The listing builds one solid part. Answer for the finished solid, in the listing's coordinates (mm). Coordinates: 2 decimals unless noted, no trailing zeros. Order: outer loops, then holes, each group sorted by start corner. A loop starts at its lowest first (then second) coordinate and runs counter-clockwise, first axis right, second up. Notation, with made-up numbers: M -9,-26.5 L 36,-26.5 A24 ccw 36,12.5 Z; hole C 52.25,17.25 d3. An arc over 180 degrees is marked long. One line per item, written item: value. Start each with the question number.
Q1. Straight lines are drawn through the part: line 1 along Z through (x, y) = (366.5, 8.25); line 2 along X through (y, z) = (10.75, -336); line 3 along Z through (x, y) = (234.5, 7). For each, find the intervals that lie inside material, in ascending order. Write a range as [from, to].
Q2. The part is cut by section C-C on x = 143.5. Give the vertices of the cut face in (y, z).
Q3. The part is cut by section B-B on z = -556. Give the vertices of the cut face in (x, y), then the cut area to 3 significant figures.
Q4. Each of these flat-tipped pins is pushed along its axis until it touches: pin 1 Ø1 at (x, y) = (110.5, 2) entering from +Z; pin 2 Ø3 at (x, y) = (250, 5) entering from +Z; pin 3 Ø2 at (x, y) = (98, 1.5) entering from -Z. Where does it stop, or does it pass through?
Q5. The part is cut by section A-A on y = 9. Give the vertices of the cut face in (x, z).
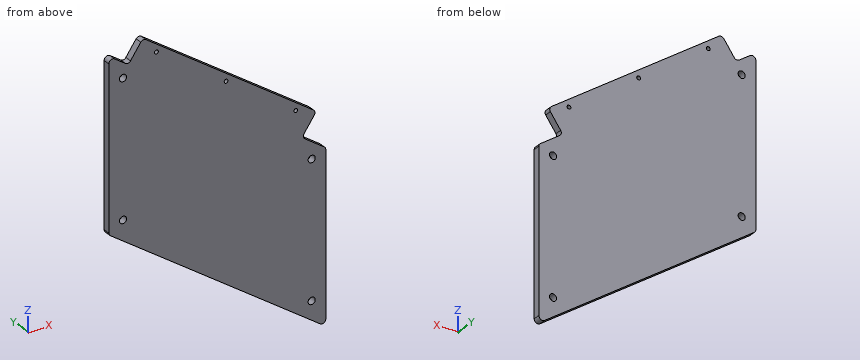
```python
from build123d import *

# Parameters (mm, degrees)
BOSS_EXTRUDE1_DEPTH = 12.7
CUT_EXTRUDE1_DEPTH  = 742.687355867
SKETCH3_R           = 3.3782
SKETCH3_R_2         = 6.35
CUT_EXTRUDE2_DEPTH  = 742.687355867
FILLET1_R           = 6.604


with BuildPart() as part:
    # Sketch1 → Boss-Extrude1 (new body)
    with BuildSketch(Plane(origin=(0, 0, 0), x_dir=(1, 0, 0), z_dir=(0, 1, 0))):
        Polygon((0, 0), (0, 359.06343047), (388.9375, 631.400399863), (388.9375, 272.336969392), align=None)
    extrude(amount=BOSS_EXTRUDE1_DEPTH)

    # Sketch2 → Cut-Extrude1 (cut, through all)
    with BuildSketch(Plane(origin=(0, 12.7, 0), x_dir=(1, 0, 0), z_dir=(0, 1, 0))):
        Polygon((35.056131737, 79.74022841), (60.988669577, 42.704726183), (0, 0), (0, 55.193660707), align=None)
        Polygon((388.9375, 327.5306301), (346.099711846, 297.535287914), (372.032249686, 260.499785687), (388.9375, 272.336969392), align=None)
    extrude(amount=-CUT_EXTRUDE1_DEPTH, mode=Mode.SUBTRACT)

    # Sketch3 → Cut-Extrude2 (cut, through all)
    with BuildSketch(Plane(origin=(0, 12.7, 0), x_dir=(1, 0, 0), z_dir=(0, 1, 0))):
        with Locations(Location((210.136591483, 160.705083027, 0), (0, 0, 270))):
            Circle(SKETCH3_R)
        with Locations(Location((334.975363032, 248.118131927, 0), (0, 0, 270))):
            Circle(SKETCH3_R)
        with Locations(Location((85.297819933, 73.292034127, 0), (0, 0, 270))):
            Circle(SKETCH3_R)
        with Locations(Location((25.4, 99.643660707, 0), (0, 0, 270))):
            Circle(SKETCH3_R_2)
        with Locations(Location((25.4, 340.943660707, 0), (0, 0, 270))):
            Circle(SKETCH3_R_2)
        with Locations(Location((363.5375, 339.300399863, 0), (0, 0, 270))):
            Circle(SKETCH3_R_2)
        with Locations(Location((363.5375, 580.600399863, 0), (0, 0, 270))):
            Circle(SKETCH3_R_2)
    extrude(amount=-CUT_EXTRUDE2_DEPTH, mode=Mode.SUBTRACT)

    # Fillet1
    fillet1_edges = [part.edges().sort_by_distance(p)[0] for p in [
        (0, 6.35, -55.193660707),
        (35.056131737, 6.35, -79.74022841),
        (60.988669577, 6.35, -42.704726183),
        (388.9375, 6.35, -327.5306301),
        (372.032249686, 6.35, -260.499785687),
        (346.099711846, 6.35, -297.535287914),
        (0, 6.35, -359.06343047),
        (388.9375, 6.35, -631.400399863),
    ]]
    fillet(fillet1_edges, radius=FILLET1_R)


solid = part.part
```
Output:
1. line 1: z = [-615.69, -586.22], [-574.98, -344.92], [-333.68, -311.82], [-268.4, -256.63]
1. line 2: x = [0, 21.41], [29.39, 358.11], [368.96, 388.94]
1. line 3: z = [-523.26, -164.2]
2. outline: M 0,-459.54 L 12.7,-459.54 L 12.7,-100.48 L 0,-100.48 Z
3. outline: M 281.25,0 L 388.94,0 L 388.94,12.7 L 281.25,12.7 Z
3. area: 1,370 mm^2
4. pin 1: stops at z = -77.02
4. pin 2: stops at z = -174
4. pin 3: stops at z = -428.38
5. outline: M 0,-355.63 A6.6 ccw 2.82,-361.04 L 378.55,-624.12 A6.6 ccw 388.94,-618.71 L 388.94,-330.97 A6.6 ccw 386.12,-325.56 L 351.51,-301.32 A6.6 cw 349.89,-292.13 L 368.24,-265.91 A6.6 ccw 366.62,-256.71 L 66.4,-46.49 A6.6 ccw 57.2,-48.11 L 38.84,-74.33 A6.6 cw 29.65,-75.95 L 10.39,-62.47 A6.6 ccw 0,-67.88 Z; hole C 25.4,-340.94 d12.7; hole C 25.4,-99.64 d12.7; hole C 85.3,-73.29 d6.76; hole C 210.14,-160.71 d6.76; hole C 334.98,-248.12 d6.76; hole C 363.54,-580.6 d12.7; hole C 363.54,-339.3 d12.7
